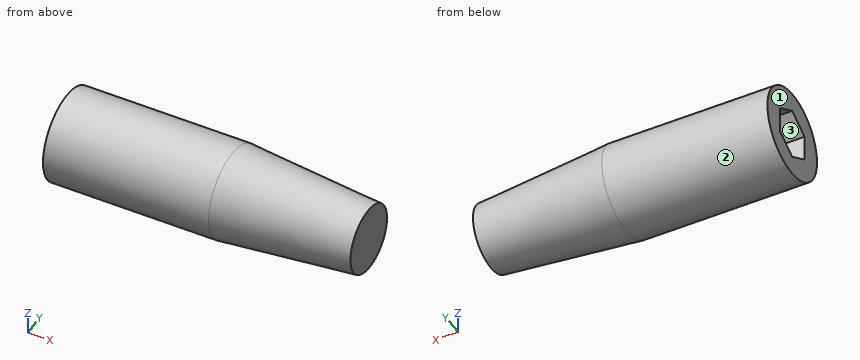
from build123d import *

# Parameters (mm, degrees)
WYTNIJ_WYCI_GNI_CIE1_DEPTH = 6


with BuildPart() as part:
    # Szkic1 → Obrót1 (revolve)
    with BuildSketch(Plane.XY, mode=Mode.PRIVATE) as obr_t1_sk:
        Polygon((0, 0), (0, 3), (11, 3), (20, 2.212602028), (20, 0), align=None)
    revolve(obr_t1_sk.sketch.rotate(Axis((0, 0, 0), (1, 0, 0)), 180), axis=Axis((0, 0, 0), (1, 0, 0)))

    # Szkic2 → Wytnij-wyciągnięcie1 (cut)
    with BuildSketch(Plane.ZY):
        Polygon((1.732050808, 0), (0.866025404, 1.5), (-0.866025404, 1.5), (-1.732050808, 0), (-0.866025404, -1.5), (0.866025404, -1.5), align=None)
    extrude(amount=-WYTNIJ_WYCI_GNI_CIE1_DEPTH, mode=Mode.SUBTRACT)


solid = part.part
Design review of the part built by this model. Coordinates are the model's own, in mm. Face numbers are marked on the shaded views. Round coordinates to 2 decimals unless told otherwise and drop trailing zeros. Order: outer loops, then holes, each group sorted by start corner. A loop starts at its lowest first (then second) coordinate and runs counter-clockwise, first axis right, second up.
1) Draft analysis for pull direction Z (two halves, no side actions). For the marked faces 1, 2 and 3, state which applies: released by +Z, released by -Z, zero draft, split by the parting line, or undercut.
The answers:
face 1: zero draft
face 2: split by the parting line
face 3: undercut
2) Consider section C-C (x = 12). State the section outline as (y, z) points.
The answers:
outline: circle Ø5.83 at (0, 0)
3) For L1, parallel to X at y = -1.05, z = -0.8; L2, parallel to Y at x = 5.5, z = -1.4; L3, parallel to Y at x = 4.5, z = 0.2, list the stretches that pass through material, from the lowest coordinate up.
The answers:
L1: x = 6 to 20
L2: y = -2.65 to -0.58, 0.58 to 2.65
L3: y = -2.99 to -1.5, 1.5 to 2.99
4) Consider section B-B (z = 0). State the section outline as (x, y) points.
The answers:
outline: (0, -3) - (11, -3) - (20, -2.21) - (20, 2.21) - (11, 3) - (0, 3) - (0, 1.5) - (6, 1.5) - (6, -1.5) - (0, -1.5) - close
5) Consider section A-A (x = 5.25). State the section outline as (y, z) points.
The answers:
outline: circle Ø6 at (0, 0); hole (-1.5, -0.87) - (0, -1.73) - (1.5, -0.87) - (1.5, 0.87) - (0, 1.73) - (-1.5, 0.87) - close
6) Clearance check with flat-ended pins moving along their axes: pin 1 Ø0.9 at (y, z) = (0.5, 0.5) entering from -X; pin 2 Ø1 at (x, y) = (15.5, -2) entering from -Z; pin 3 Ø1 at (x, y) = (12.5, 1) entering from +Z (3 decimals). State where each tip first meets the part, or that it passes through.
The answers:
pin 1: stops at x = 6
pin 2: stops at z = -2.14
pin 3: stops at z = 2.835
7) Consider section D-D (x = 15). State the section outline as (y, z) points, plus the area to 3 significant figures.
The answers:
outline: circle Ø5.3 at (0, 0)
area: 22.1 mm2
